Geometry: final body of the model. Coordinates: model frame, mm. Face numbers are marked on the shaded views. A direction names the side the tool comes from. Give positions to 0.01 mm unless a question says otherwise; leave off trailing zeros. Write each loop counter-clockwise with the first axis right and the second up, starting at its lowest first coordinate (ties: lowest second). Pieces come first, ordered by that corner, then holes. Notation, with made-up numbers: M -33,-36 L 23,-36 A23 ccw 23,-12 Z; hole C 67,4 d2. An arc over 180 degrees is marked long. Answer as a JSON object with one key per item and string values.
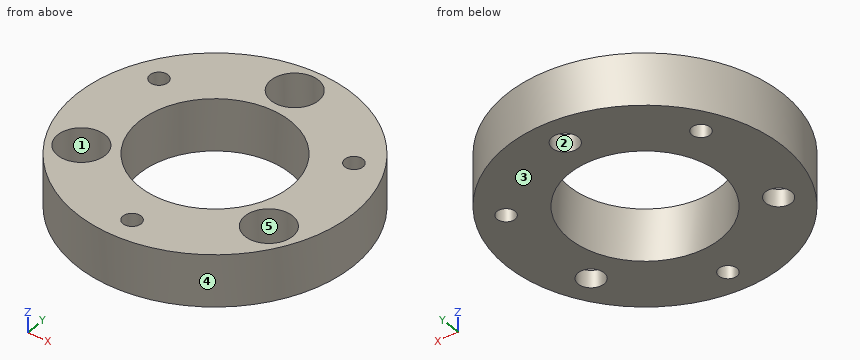
from build123d import *

# Parameters (mm, degrees)
SKETCH_R     = 32
SKETCH_R_2   = 2.1
SKETCH_R_3   = 3
SKETCH_R_4   = 17.5
PAD_DEPTH    = 12
SKETCH001_R  = 5.5
POCKET_DEPTH = 8


with BuildPart() as part:
    # Sketch → Pad (new body)
    with BuildSketch(Plane.XY):
        Circle(SKETCH_R)
        with Locations((0, -26)):
            Circle(SKETCH_R_2, mode=Mode.SUBTRACT)
        with Locations((-22.51666, 13)):
            Circle(SKETCH_R_2, mode=Mode.SUBTRACT)
        with Locations((22.51666, 13)):
            Circle(SKETCH_R_2, mode=Mode.SUBTRACT)
        with Locations((0, 25)):
            Circle(SKETCH_R_3, mode=Mode.SUBTRACT)
        with Locations((-21.650635, -12.5)):
            Circle(SKETCH_R_3, mode=Mode.SUBTRACT)
        with Locations((21.650635, -12.5)):
            Circle(SKETCH_R_3, mode=Mode.SUBTRACT)
        Circle(SKETCH_R_4, mode=Mode.SUBTRACT)
    extrude(amount=PAD_DEPTH)

    # Sketch001 (on Face10 of Pad) → Pocket (cut)
    with BuildSketch(Plane.XY.offset(12)):
        with Locations((0, 25)):
            Circle(SKETCH001_R)
        with Locations((-21.650635, -12.5)):
            Circle(SKETCH001_R)
        with Locations((21.650635, -12.5)):
            Circle(SKETCH001_R)
    extrude(amount=-POCKET_DEPTH, mode=Mode.SUBTRACT)


solid = part.part
1) Cut plane A-A on y = 0. Return loops of the section in (x, z), and give its area (3 significant figures).
Geometry check:
{"outline": "M -32,0 L -17.5,0 L -17.5,12 L -32,12 Z; M 17.5,0 L 32,0 L 32,12 L 17.5,12 Z", "area": "348 mm2"}
2) Contact query for flat-ended pins moving along their axis: P1, Ø1, axis at x = 0, z = 8.5, coming from the -Y side; P2, Ø3.5, axis at x = 0, y = -26, coming from the -Z side; P3, Ø2, axis at y = -12, z = 7, coming from the +X side; P4, Ø8, axis at x = 21.65, y = -12.5, coming from the +Z side. Output: stop coordinate, or through.
Geometry check:
{"P1": "stops at y = -32", "P2": "passes through", "P3": "stops at x = 30.05", "P4": "stops at z = 4"}
3) Cut plane D-D on x = 7. Return loops of the section in (y, z).
Geometry check:
{"outline": "M -31.22,0 L -16.04,0 L -16.04,12 L -31.22,12 Z; M 16.04,0 L 31.22,0 L 31.22,12 L 16.04,12 Z"}
4) Line query: line 1 (Y direction, x = 0, z = 2.5); line 2 (Y direction, x = -22, z = 4.75); line 3 (X direction, y = -9, z = 9.75). Output: solid intervals per line, ascending. Write a range as from..to.
Geometry check:
{"line 1": "y = -32..-28.1, -23.9..-17.5, 17.5..22, 28..32", "line 2": "y = -23.24..-17.99, -7.01..10.96, 15.04..23.24", "line 3": "x = -30.71..-25.89, -17.41..-15.01, 15.01..17.41, 25.89..30.71"}
5) Set-up query: the marked faces 1 and 2. Return all of +Z, -Z, +X, -X, +Y, -Y with unobstructed straight access to the full face (end or side cutting, diameter ignored); none if empty.
Geometry check:
{"face 1": "+Z", "face 2": "+Z, -Z"}
6) Pull-direction query (X, two-part tool) for the marked faces 3, 4 and 5; classes: pulls with the +X half, pulls with the -X half, needs draft (parallel to the pull), parting line crosses it, or undercut.
Geometry check:
{"face 3": "needs draft", "face 4": "parting line crosses it", "face 5": "undercut"}
7) Cut plane C-C on x = 0. Return loops of the section in (y, z).
Geometry check:
{"outline": "M -32,0 L -28.1,0 L -28.1,12 L -32,12 Z; M -23.9,0 L -17.5,0 L -17.5,12 L -23.9,12 Z; M 17.5,0 L 22,0 L 22,4 L 19.5,4 L 19.5,12 L 17.5,12 Z; M 28,0 L 32,0 L 32,12 L 30.5,12 L 30.5,4 L 28,4 Z"}
8) Cut plane B-B on z = 5.75. Return loops of the section in (x, y), and give its area (3 significant figures).
Geometry check:
{"outline": "C 0,0 d64; hole C -21.65,-12.5 d11; hole C -22.52,13 d4.2; hole C 0,0 d35; hole C 0,25 d11; hole C 0,-26 d4.2; hole C 21.65,-12.5 d11; hole C 22.52,13 d4.2", "area": "1,930 mm2"}
